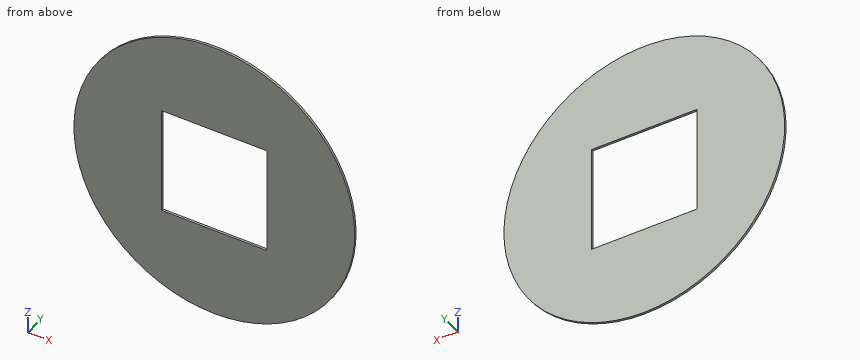
from build123d import *

# Parameters (mm, degrees)
SKETCH1_W           = 40
SKETCH1_H           = 1.57
BOSS_EXTRUDE1_START = -1.57
SKETCH2_R           = 60
SKETCH2_W           = 75
SKETCH2_H           = 75
BOSS_EXTRUDE1_DEPTH = 1.57


with BuildPart() as part:
    # Sketch1 → Revolve1 (revolve)
    with BuildSketch(Plane.XY, mode=Mode.PRIVATE) as revolve1_sk:
        with Locations((-80, 0)):
            Rectangle(SKETCH1_W, SKETCH1_H)
    revolve(revolve1_sk.sketch.rotate(Axis((0, -200069.047495165, 0), (0, 1, 0)), 270), axis=Axis((0, -200069.047495165, 0), (0, 1, 0)))

    # Sketch2 → Boss-Extrude1 (add)
    with BuildSketch(Plane(origin=(0, 0.785, 0), x_dir=(1, 0, 0), z_dir=(0, 1, 0)).offset(BOSS_EXTRUDE1_START)):
        Circle(SKETCH2_R)
        Rectangle(SKETCH2_W, SKETCH2_H, mode=Mode.SUBTRACT)
    extrude(amount=BOSS_EXTRUDE1_DEPTH)


solid = part.part
The model under review builds one solid part; all positions refer to its coordinate system, in mm. Round coordinates to 2 decimals unless told otherwise and drop trailing zeros. Order: outer loops, then holes, each group sorted by start corner. A loop starts at its lowest first (then second) coordinate and runs counter-clockwise, first axis right, second up. Notation, with made-up numbers: (40, 75) -> (78, 75) arc R5 cw to (78, 80) -> close; hole circle Ø7 at (8.5, 21.25). An arc over 180 degrees is marked (long way). Use CSV: the item, a comma, the result in double quotes. Start each with the question number.
(1) Consider section C-C on y = 0.5. Write out the cut boundary in (x, z).
(2) Consider section D-D on x = 46. Write out the cut boundary in (y, z) (3 decimals).
(3) Insertion check: pin 1 (0.5 mm diameter, centred on y = 0, z = -14, fed in from +X); pin 2 (0.5 mm diameter, centred on x = 10, y = -0.5, fed in from -Z). Each pin has a flat end and moves straight along its axis. Give the tip position at first contact, or say it passes through.
(4) Consider section B-B on x = 0. Write out the cut boundary in (y, z) (3 decimals), and give its area (3 significant figures).
(5) Wall thickness on probe 1 along X at (y, z) = (0.05, 2.5); probe 2 along X at (y, z) = (-0.45, 14); probe 3 along Z at (x, y) = (35, 0.2): over which ranges is each line inside the solid? List them lowest first. Write a range as from..to.
(6) Consider section A-A on z = 0. Write out the cut boundary in (x, y) (3 decimals).
Responses:
1,outline,"circle Ø200 at (0, 0); hole (-37.5, -37.5) -> (37.5, -37.5) -> (37.5, 37.5) -> (-37.5, 37.5) -> close"
2,outline,"(-0.785, -88.792) -> (0.785, -88.792) -> (0.785, 88.792) -> (-0.785, 88.792) -> close"
3,pin 1,"x = 99.05"
3,pin 2,"z = -99.52"
4,outline,"(-0.785, -100) -> (0.785, -100) -> (0.785, -37.5) -> (-0.785, -37.5) -> close; (-0.785, 37.5) -> (0.785, 37.5) -> (0.785, 100) -> (-0.785, 100) -> close"
4,area,"196 mm²"
5,probe 1,"-99.97..-37.5, 37.5..99.97"
5,probe 2,"-99.02..-37.5, 37.5..99.02"
5,probe 3,"-93.67..-37.5, 37.5..93.67"
6,outline,"(-100, -0.785) -> (-37.5, -0.785) -> (-37.5, 0.785) -> (-100, 0.785) -> close; (37.5, -0.785) -> (100, -0.785) -> (100, 0.785) -> (37.5, 0.785) -> close"
